from build123d import *

# Parameters (mm, degrees)
BOX010_W          = 3
BOX010_H          = 34
BOX010_DEPTH      = 15
BOX016_W          = 3
BOX016_H          = 34
BOX016_DEPTH      = 15
BOX013_W          = 3
BOX013_H          = 34
BOX013_DEPTH      = 15
BOX015_W          = 3
BOX015_H          = 34
BOX015_DEPTH      = 15
BOX012_W          = 3
BOX012_H          = 34
BOX012_DEPTH      = 15
BOX014_W          = 3
BOX014_H          = 34
BOX014_DEPTH      = 15
BOX011_W          = 3
BOX011_H          = 34
BOX011_DEPTH      = 15
BOX009_W          = 3
BOX009_H          = 34
BOX009_DEPTH      = 15
CYLINDER015_R     = 3.1
CYLINDER015_DEPTH = 3
CYLINDER017_R     = 3.1
CYLINDER017_DEPTH = 3
CYLINDER016_R     = 3.1
CYLINDER016_DEPTH = 3
CYLINDER014_R     = 3.1
CYLINDER014_DEPTH = 3
CYLINDER010_R     = 1.7
CYLINDER010_DEPTH = 10
CYLINDER013_R     = 1.7
CYLINDER013_DEPTH = 10
CYLINDER011_R     = 1.7
CYLINDER011_DEPTH = 10
CYLINDER012_R     = 1.7
CYLINDER012_DEPTH = 10
BOX008_W          = 71
BOX008_H          = 45
BOX008_DEPTH      = 5
BOX007_W          = 76
BOX007_H          = 50
BOX007_DEPTH      = 5
FILLET006_R       = 4


with BuildPart() as cubo001:
    # Box010 → Box010 (new body)
    with BuildSketch(Plane(origin=(16, 7, 46), x_dir=(1, 0, 0), z_dir=(0, 0, 1))):
        with Locations((1.5, 17)):
            Rectangle(BOX010_W, BOX010_H)
    extrude(amount=BOX010_DEPTH)


with BuildPart() as cubo007:
    # Box016 → Box016 (new body)
    with BuildSketch(Plane(origin=(64, 7, 46), x_dir=(1, 0, 0), z_dir=(0, 0, 1))):
        with Locations((1.5, 17)):
            Rectangle(BOX016_W, BOX016_H)
    extrude(amount=BOX016_DEPTH)


with BuildPart() as cubo004:
    # Box013 → Box013 (new body)
    with BuildSketch(Plane(origin=(40, 7, 46), x_dir=(1, 0, 0), z_dir=(0, 0, 1))):
        with Locations((1.5, 17)):
            Rectangle(BOX013_W, BOX013_H)
    extrude(amount=BOX013_DEPTH)


with BuildPart() as cubo006:
    # Box015 → Box015 (new body)
    with BuildSketch(Plane(origin=(56, 7, 46), x_dir=(1, 0, 0), z_dir=(0, 0, 1))):
        with Locations((1.5, 17)):
            Rectangle(BOX015_W, BOX015_H)
    extrude(amount=BOX015_DEPTH)


with BuildPart() as cubo003:
    # Box012 → Box012 (new body)
    with BuildSketch(Plane(origin=(32, 7, 46), x_dir=(1, 0, 0), z_dir=(0, 0, 1))):
        with Locations((1.5, 17)):
            Rectangle(BOX012_W, BOX012_H)
    extrude(amount=BOX012_DEPTH)


with BuildPart() as cubo005:
    # Box014 → Box014 (new body)
    with BuildSketch(Plane(origin=(48, 7, 46), x_dir=(1, 0, 0), z_dir=(0, 0, 1))):
        with Locations((1.5, 17)):
            Rectangle(BOX014_W, BOX014_H)
    extrude(amount=BOX014_DEPTH)


with BuildPart() as cubo002:
    # Box011 → Box011 (new body)
    with BuildSketch(Plane(origin=(24, 7, 46), x_dir=(1, 0, 0), z_dir=(0, 0, 1))):
        with Locations((1.5, 17)):
            Rectangle(BOX011_W, BOX011_H)
    extrude(amount=BOX011_DEPTH)


with BuildPart() as fusion006:
    # Box009 → Box009 (new body)
    with BuildSketch(Plane(origin=(8, 7, 46), x_dir=(1, 0, 0), z_dir=(0, 0, 1))):
        with Locations((1.5, 17)):
            Rectangle(BOX009_W, BOX009_H)
    extrude(amount=BOX009_DEPTH)

    # Fusion006: union Cubo001, Cubo007, Cubo004, Cubo006, Cubo003, Cubo005, Cubo002
    add(cubo001.part)
    add(cubo007.part)
    add(cubo004.part)
    add(cubo006.part)
    add(cubo003.part)
    add(cubo005.part)
    add(cubo002.part)


with BuildPart() as obj1:
    # Cylinder015 → Cylinder015 (new body)
    with BuildSketch(Plane(origin=(71, 3, 40), x_dir=(1, 0, 0), z_dir=(0, 0, 1))):
        Circle(CYLINDER015_R)
    extrude(amount=CYLINDER015_DEPTH)


with BuildPart() as obj2:
    # Cylinder017 → Cylinder017 (new body)
    with BuildSketch(Plane(origin=(3, 45, 40), x_dir=(1, 0, 0), z_dir=(0, 0, 1))):
        Circle(CYLINDER017_R)
    extrude(amount=CYLINDER017_DEPTH)


with BuildPart() as obj3:
    # Cylinder016 → Cylinder016 (new body)
    with BuildSketch(Plane(origin=(71, 45, 40), x_dir=(1, 0, 0), z_dir=(0, 0, 1))):
        Circle(CYLINDER016_R)
    extrude(amount=CYLINDER016_DEPTH)


with BuildPart() as obj4:
    # Cylinder014 → Cylinder014 (new body)
    with BuildSketch(Plane(origin=(3, 3, 40), x_dir=(1, 0, 0), z_dir=(0, 0, 1))):
        Circle(CYLINDER014_R)
    extrude(amount=CYLINDER014_DEPTH)

    # Fusion005: union obj1, obj2, obj3
    add(obj1.part)
    add(obj2.part)
    add(obj3.part)


with BuildPart() as obj4_1:
    # Fusion005 placement: moved
    add(obj4.part.moved(Location((0, 0, 12))))


with BuildPart() as obj5:
    # Cylinder010 → Cylinder010 (new body)
    with BuildSketch(Plane(origin=(71, 3, 40), x_dir=(1, 0, 0), z_dir=(0, 0, 1))):
        Circle(CYLINDER010_R)
    extrude(amount=CYLINDER010_DEPTH)


with BuildPart() as obj6:
    # Cylinder013 → Cylinder013 (new body)
    with BuildSketch(Plane(origin=(3, 45, 40), x_dir=(1, 0, 0), z_dir=(0, 0, 1))):
        Circle(CYLINDER013_R)
    extrude(amount=CYLINDER013_DEPTH)


with BuildPart() as obj7:
    # Cylinder011 → Cylinder011 (new body)
    with BuildSketch(Plane(origin=(71, 45, 40), x_dir=(1, 0, 0), z_dir=(0, 0, 1))):
        Circle(CYLINDER011_R)
    extrude(amount=CYLINDER011_DEPTH)


with BuildPart() as obj8:
    # Cylinder012 → Cylinder012 (new body)
    with BuildSketch(Plane(origin=(3, 3, 40), x_dir=(1, 0, 0), z_dir=(0, 0, 1))):
        Circle(CYLINDER012_R)
    extrude(amount=CYLINDER012_DEPTH)

    # Fusion004: union obj5, obj6, obj7
    add(obj5.part)
    add(obj6.part)
    add(obj7.part)


with BuildPart() as obj8_1:
    # Fusion004 placement: moved
    add(obj8.part.moved(Location((0, 0, 6))))


with BuildPart() as vaciado_interior001:
    # Box008 → Box008 (new body)
    with BuildSketch(Plane(origin=(1.5, 1.5, 46.5), x_dir=(1, 0, 0), z_dir=(0, 0, 1))):
        with Locations((35.5, 22.5)):
            Rectangle(BOX008_W, BOX008_H)
    extrude(amount=BOX008_DEPTH)


with BuildPart() as obj9:
    # Box007 → Box007 (new body)
    with BuildSketch(Plane(origin=(-1, -1, 50), x_dir=(1, 0, 0), z_dir=(0, 0, 1))):
        with Locations((38, 25)):
            Rectangle(BOX007_W, BOX007_H)
    extrude(amount=BOX007_DEPTH)

    # Cut006: cut vaciado interior001
    add(vaciado_interior001.part, mode=Mode.SUBTRACT)

    # Fillet006
    fillet006_edges = [obj9.edges().sort_by_distance(p)[0] for p in [
        (-1, -1, 52.5),
        (-1, 49, 52.5),
        (75, -1, 52.5),
        (75, 49, 52.5),
    ]]
    fillet(fillet006_edges, radius=FILLET006_R)

    # Cut007: cut obj8
    add(obj8_1.part, mode=Mode.SUBTRACT)

    # Cut008: cut obj4
    add(obj4_1.part, mode=Mode.SUBTRACT)

    # Cut009: cut Fusion006
    add(fusion006.part, mode=Mode.SUBTRACT)


with BuildPart() as obj9_1:
    # Cut009 placement: moved
    add(obj9.part.moved(Location((0, 0, 32))))


solid = obj9_1.part
Geometry check sheet. Reference: the model listing, model coordinates, mm. A direction names the side the tool comes from. Give positions to 0.01 mm unless a question says otherwise; leave off trailing zeros. Write each loop counter-clockwise with the first axis right and the second up, starting at its lowest first coordinate (ties: lowest second). Pieces come first, ordered by that corner, then holes.
1) Thickness scan on line 1 (Y direction, x = 71, z = 85); line 2 (Y direction, x = 10.5, z = 84.35); line 3 (Y direction, x = 8, z = 82.7). Record the ranges inside material, lowest first.
Values follow:
line 1: y = -1 to -0.1, 6.1 to 41.9, 48.1 to 49
line 2: y = -1 to 7, 41 to 49
line 3: y = -1 to 1.5, 46.5 to 49
2) Release check for a two-part mould opening along Y. For faces 6 (the face through (36, 24, 87)), 7 (the face through (1.5, 24, 83)), 8 (the face through (37, -1, 84)) record: released by +Y, released by -Y, zero draft, split by the parting line, or undercut.
Values follow:
face 6: zero draft
face 7: undercut
face 8: released by -Y
3) Cross-section at B-B (y = 38). Count the separate pieces of the cut face and the enclosed holes in it, plus the area to 4 significant figures.
Values follow:
separate pieces: 9
enclosed holes: 0
area: 189.5 mm2
4) Set-up check for faces 1 (the face through (72.33, 43.67, 84)), 2 (the face through (25, 7, 85)), 3 (the face through (37, 49, 84)), 4 (the face through (37, 24, 83.5)), 5 (the face through (75, 24, 84)): record each of +Z, -Z, +X, -X, +Y, -Y from which the full face is reachable in a straight line by a thin tool's end or side.
Values follow:
face 1: +Z
face 2: +Z, -Z
face 3: +Z, -Z, +X, -X, +Y
face 4: -Z
face 5: +Z, -Z, +X, +Y, -Y
5) Cross-section at A-A (x = 62). Record the boundary of the cut face in (y, z).
Values follow:
outline: (-1, 82) - (1.5, 82) - (1.5, 83.5) - (46.5, 83.5) - (46.5, 82) - (49, 82) - (49, 87) - (-1, 87) - close
6) Go/stop test with flat-tipped pins: pin 1 Ø2 at (x, y) = (71, 3) entering from -Z; pin 2 Ø5.5 at (x, y) = (3, 3) entering from +Z; pin 3 Ø0.6 at (y, z) = (46.5, 82.5) entering from +X. Record where each tip stops, or that it passes through.
Values follow:
pin 1: passes through
pin 2: stops at z = 84
pin 3: stops at x = 74.82
